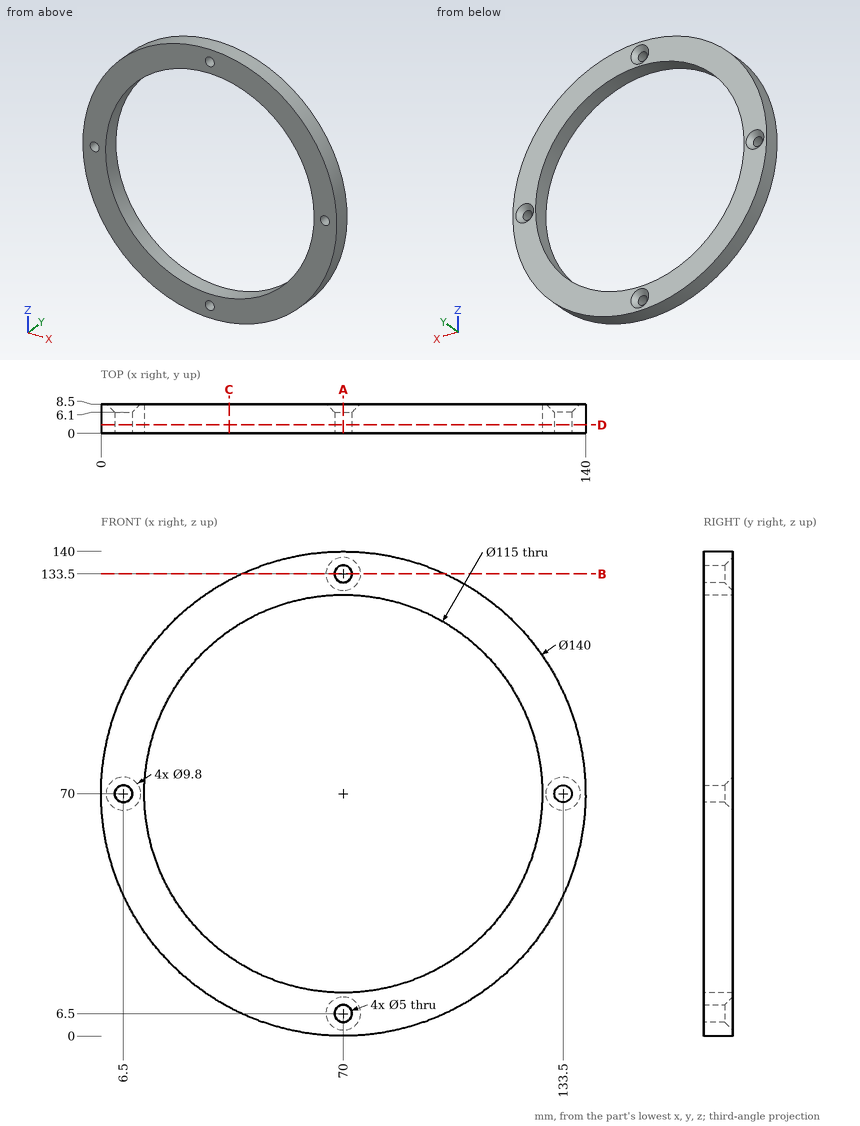
Print and shaded views of the part. All mm, measured from the part's lowest x, y and z. Give positions to 0.01 mm unless a question says otherwise; leave off trailing zeros. Write each loop counter-clockwise with the first axis right and the second up, starting at its lowest first coordinate (ties: lowest second). Pieces come first, ordered by that corner, then holes. Notation, with made-up numbers: (-22, -21.5) -> (-9, -21.5) arc R28 cw to (-9, 1.5) -> close; hole circle Ø1 at (71.5, -4.5). An arc over 180 degrees is marked (long way). Use CSV: the item, a comma, the result in double quotes. Start each with the question number.
1) Pin check, flat tips, straight feed: P1, Ø2, axis at x = 21.5, y = 6.5, coming from the -Z side; P2, Ø5, axis at x = 41.5, y = 2, coming from the -Z side; P3, Ø1, axis at y = 5, z = 123, coming from the +X side; P4, Ø3, axis at x = 6.5, z = 70, coming from the -Y side. Stop position of each tip, or through.
2) Cut at B-B on z = 133.5. List the corners of the cut face in (x, y), plus the area to 3 significant figures.
3) Cut at A-A on x = 70. List the corners of the cut face in (y, z).
4) Cut at D-D on y = 2.5. List the corners of the cut face in (x, z), plus the area to 3 significant figures.
5) Cut at C-C on x = 37. List the corners of the cut face in (y, z), plus the area to 3 significant figures.
6) Drill centre lines: L1, parallel to X at y = 2, z = 70; L2, parallel to Z at x = 64, y = 2.75; L3, parallel to X at y = 2.75, z = 109.5. Where is each one in solid material? Low to high.
Final values:
1,P1,"stops at z = 18.58"
1,P2,"stops at z = 5.01"
1,P3,"stops at x = 116.3"
1,P4,"passes through"
2,outline,"(40.54, 0) -> (67.5, 0) -> (67.5, 6.1) -> (65.1, 8.5) -> (40.54, 8.5) -> close; (72.5, 0) -> (99.46, 0) -> (99.46, 8.5) -> (74.9, 8.5) -> (72.5, 6.1) -> close"
2,area,"453 mm2"
3,outline,"(0, 0) -> (8.5, 0) -> (8.5, 1.6) -> (6.1, 4) -> (0, 4) -> close; (0, 9) -> (6.1, 9) -> (8.5, 11.4) -> (8.5, 12.5) -> (0, 12.5) -> close; (0, 127.5) -> (8.5, 127.5) -> (8.5, 128.6) -> (6.1, 131) -> (0, 131) -> close; (0, 136) -> (6.1, 136) -> (8.5, 138.4) -> (8.5, 140) -> (0, 140) -> close"
4,outline,"circle Ø140 at (70, 70); hole circle Ø5 at (6.5, 70); hole circle Ø115 at (70, 70); hole circle Ø5 at (70, 6.5); hole circle Ø5 at (70, 133.5); hole circle Ø5 at (133.5, 70)"
4,area,"4,930 mm2"
5,outline,"(0, 8.27) -> (8.5, 8.27) -> (8.5, 22.91) -> (0, 22.91) -> close; (0, 117.09) -> (8.5, 117.09) -> (8.5, 131.73) -> (0, 131.73) -> close"
5,area,"249 mm2"
6,L1,"x = 0 to 4, 9 to 12.5, 127.5 to 131, 136 to 140"
6,L2,"z = 0.26 to 12.81, 127.19 to 139.74"
6,L3,"x = 12.21 to 28.21, 111.79 to 127.79"
